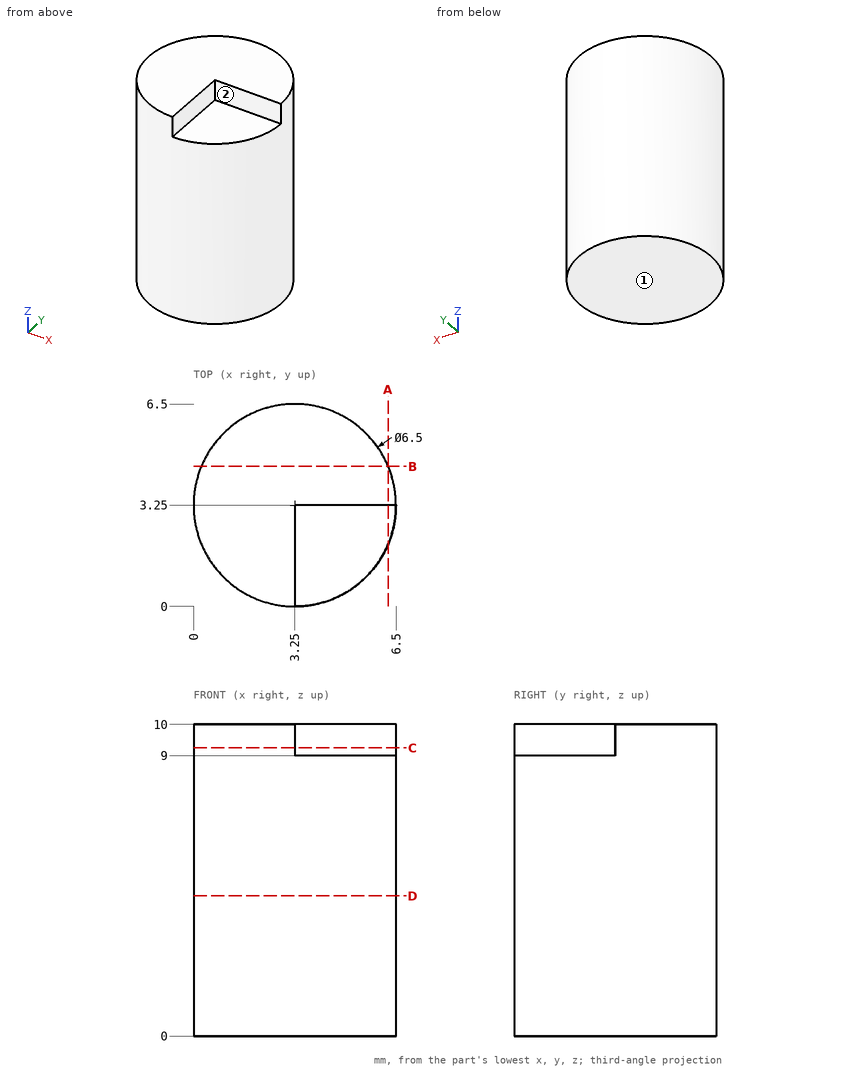
Verification items for this drawing (mm, ordinates from the low corner). A direction names the side the tool comes from. Round coordinates to 2 decimals unless told otherwise and drop trailing zeros. Order: outer loops, then holes, each group sorted by start corner. A loop starts at its lowest first (then second) coordinate and runs counter-clockwise, first axis right, second up. Notation, with made-up numbers: (-32, 84) - (27, 84) arc R24 ccw to (27, 110) - close; hole circle Ø9 at (18, 61.5). An arc over 180 degrees is marked (long way). Use CSV: the item, a comma, the result in double quotes.
(1) Gauge pin test, flat ends, axial feed: pin 1 Ø0.5 at (x, z) = (4, 9.5) entering from -Y; pin 2 Ø0.8 at (y, z) = (1, 9.5) entering from +X; pin 3 Ø1 at (y, z) = (5, 6) entering from -X. Record the tip position at first contact, or that the pin passes through.
Entries:
pin 1,"y = 3.25"
pin 2,"x = 3.25"
pin 3,"x = 0.25"
(2) Section check C-C on z = 9.25. Record the boundary of the cut face in (x, y).
Entries:
outline,"(3.25, 0) - (3.25, 3.25) - (6.5, 3.25) arc R3.25 ccw (long way) to start"
(3) Section check A-A on x = 6.25. Record the boundary of the cut face in (y, z).
Entries:
outline,"(2, 0) - (4.5, 0) - (4.5, 10) - (3.25, 10) - (3.25, 9) - (2, 9) - close"
(4) Section check B-B on y = 4.5. Record the boundary of the cut face in (x, z), and give its area (3 significant figures).
Entries:
outline,"(0.25, 0) - (6.25, 0) - (6.25, 10) - (0.25, 10) - close"
area,"60.0 mm^2"
(5) Thickness scan on probe 1 along Z at (x, y) = (3.5, 2.25); probe 2 along Y at (x, z) = (0.75, 2.75); probe 3 along X at (y, z) = (1.25, 8). Record the ranges inside material, lowest first. Write a range as from..to.
Entries:
probe 1,"0..9"
probe 2,"1.17..5.33"
probe 3,"0.69..5.81"
(6) Section check D-D on z = 4.5. Record the boundary of the cut face in (x, y).
Entries:
outline,"circle Ø6.5 at (3.25, 3.25)"
(7) Access from +Z, -Z, +X, -X, +Y, -Y to the whole of each face (thin tool, end or side, straight path). Record for the marked faces 1 and 2.
Entries:
face 1,"-Z, +X, -X, +Y, -Y"
face 2,"+Z, +X, -Y"
